Input: part model. Units: mm. Frame: model coordinates. Face numbers are marked on the shaded views. Coordinates: 2 decimals unless noted, no trailing zeros. Loops run counter-clockwise (first coordinate to the right, second up) from the corner with the lowest first, then second, coordinate; pieces in that order, holes last. Notation, with made-up numbers: (61, 3) - (84, 3) arc R9 cw to (84, 8) - close; hole circle Ø8 at (86, 24.25). An arc over 180 degrees is marked (long way). Use one line per item in the form item = value.
from build123d import *

# Parameters (mm, degrees)
SKETCH1_R           = 6.5
BOSS_EXTRUDE1_DEPTH = 4.84
CHAMFER1_SIZE       = 1
CHAMFER2_SIZE       = 1.5


with BuildPart() as part:
    # Sketch1 → Boss-Extrude1 (new body)
    with BuildSketch(Plane.XY):
        Polygon((5.138417396, 8.9), (-5.138417396, 8.9), (-10.276834792, 0), (-5.138417396, -8.9), (5.138417396, -8.9), (10.276834792, 0), align=None)
        Circle(SKETCH1_R, mode=Mode.SUBTRACT)
    extrude(amount=BOSS_EXTRUDE1_DEPTH)

    # Chamfer1
    chamfer1_edges = [part.edges().sort_by_distance(p)[0] for p in [
        (10.276834792, 0, 2.42),
        (5.138417396, -8.9, 2.42),
        (-5.138417396, -8.9, 2.42),
        (-10.276834792, 0, 2.42),
        (-5.138417396, 8.9, 2.42),
        (5.138417396, 8.9, 2.42),
    ]]
    chamfer(chamfer1_edges, length=CHAMFER1_SIZE)

    # Chamfer2
    chamfer2_edges = [part.edges().sort_by_distance(p)[0] for p in [
        (4.888417396, 8.466987298, 0),
        (9.776834792, 0, 0),
        (-4.888417396, 8.466987298, 0),
        (-9.776834792, 0, 0),
        (-4.888417396, -8.466987298, 0),
        (4.888417396, -8.466987298, 0),
    ]]
    chamfer(chamfer2_edges, length=CHAMFER2_SIZE)


solid = part.part
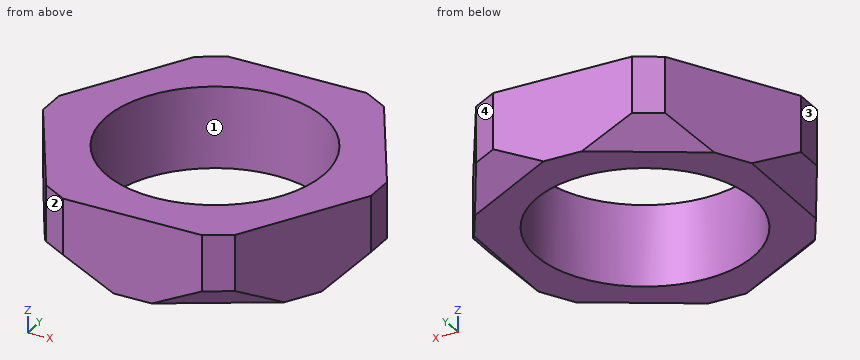
Q1. Cut plane C-C, the plane x = 0. Return loops of the section in (y, z).
Check values:
outline = (-8.9, 0) - (-6.5, 0) - (-6.5, 4.84) - (-8.9, 4.84) - close; (6.5, 0) - (8.9, 0) - (8.9, 4.84) - (6.5, 4.84) - close
Q2. Cut plane B-B, the plane y = 0. Return loops of the section in (x, z), then the cut area to 3 significant figures.
Check values:
outline = (-9.78, 1.5) - (-8.28, 0) - (-6.5, 0) - (-6.5, 4.84) - (-9.78, 4.84) - close; (6.5, 0) - (8.28, 0) - (9.78, 1.5) - (9.78, 4.84) - (6.5, 4.84) - close
area = 29.5 mm²
Q3. Ray query, line 1 along Y through (x, z) = (0, 2); line 2 along X through (y, z) = (-6, 2.7); line 3 along X through (y, z) = (0.5, 3.9). Return the intervals inside material, ascending. Write a range as [from, to].
Check values:
line_1 = [-8.9, -6.5], [6.5, 8.9]
line_2 = [-6.81, -2.5], [2.5, 6.81]
line_3 = [-9.78, -6.48], [6.48, 9.78]
Q4. First-contact query: P1, Ø1.5, axis at x = 2.5, y = 5.5, coming from the -Z side. Flat tip, straight axial feed; report the tip coordinate or a pass-through.
Check values:
P1 = 0
Q5. Pull-direction query (Y, two-part tool) for the marked faces 1, 2, 3 and 4; classes: pulls with the +Y half, pulls with the -Y half, needs draft (parallel to the pull), parting line crosses it, or undercut.
Check values:
face_1 = undercut
face_2 = pulls with the -Y half
face_3 = needs draft
face_4 = pulls with the +Y half
Q6. Cut plane A-A, the plane z = 4.35. Return loops of the section in (x, y).
Check values:
outline = (-9.78, -0.87) - (-5.64, -8.03) - (-4.14, -8.9) - (4.14, -8.9) - (5.64, -8.03) - (9.78, -0.87) - (9.78, 0.87) - (5.64, 8.03) - (4.14, 8.9) - (-4.14, 8.9) - (-5.64, 8.03) - (-9.78, 0.87) - close; hole circle Ø13 at (0, 0)
Q7. Cut plane D-D, the plane y = -6.75. Return loops of the section in (x, z), then the cut area to 3 significant figures.
Check values:
outline = (-6.38, 0.76) - (-4.86, 0) - (4.86, 0) - (6.38, 0.76) - (6.38, 4.84) - (-6.38, 4.84) - close
area = 60.6 mm²
